Verification items for the finished model (mm, model axes). Face numbers are marked on the shaded views. A direction names the side the tool comes from. Coordinates: 2 decimals unless noted, no trailing zeros. Loops run counter-clockwise (first coordinate to the right, second up) from the corner with the lowest first, then second, coordinate; pieces in that order, holes last.
Q1. Sectioned sample at B-B (y = 155.5). Enter the section's corners in (x, z).
Q2. Mould release check, pull along X, two halves, no side actions. Record for the marked faces 3 and 4: +X half, -X half, draft (parallel to the pull), parting line (faces both ways), or undercut.
Q3. Sectioned sample at A-A (x = 57). Enter the section's corners in (y, z), then the cut area to 3 significant figures.
Q4. Material ranges on probe 1 along X at (y, z) = (9, 7.5); probe 2 along Y at (x, z) = (20, 3.75); probe 3 along Y at (x, z) = (79, 9), recorded low to high.
Q5. Go/stop test with flat-tipped pins: P1, Ø7.5, axis at x = 66, z = 5, coming from the +Y side; P2, Ø4.5, axis at x = 130, z = 7.5, coming from the +Y side; P3, Ø6, axis at x = 80, z = 7.5, coming from the +Y side. Record where each tip stops, or that it passes through.
Q6. Access from +Z, -Z, +X, -X, +Y, -Y to the whole of each face (thin tool, end or side, straight path). Record for the marked faces 1 and 2.
Q7. Sectioned sample at C-C (y = 178). Enter the section's corners in (x, z), then the cut area to 3 significant figures.
```python
from build123d import *

# Parameters (mm, degrees)
EXTRUDE_1_DEPTH        = 15
CUT_EXTRUDE_1_DEPTH    = 267.118858915
FILLET_1_R             = 10
PATTERN_LINEAR_1_COUNT = 3
PATTERN_LINEAR_1_PITCH = 50
PATTERN_LINEAR_2_COUNT = 3
PATTERN_LINEAR_2_PITCH = 80
HOLE_WIZARD_M6_3_D     = 5


with BuildPart() as part:
    # 草图1 → 凸台-拉伸1 (new body)
    with BuildSketch(Plane.XY):
        Polygon((0, 0), (163.629943485, 0), (163.629943485, 94.33), (0, 209.331050409), align=None)
    extrude(amount=EXTRUDE_1_DEPTH)

    # 草图2 → 切除-拉伸1 (cut, through all)
    with BuildSketch(Plane.XY.offset(15)):
        Polygon((25, 161.2040017), (25, 25), (138.629943485, 25), (138.629943485, 81.343539854), align=None)
    extrude(amount=-CUT_EXTRUDE_1_DEPTH, mode=Mode.SUBTRACT)

    # 圆角1
    fillet_1_edges = [part.edges().sort_by_distance(p)[0] for p in [
        (25, 161.2040017, 7.5),
        (138.629943485, 81.343539854, 7.5),
        (138.629943485, 25, 7.5),
        (25, 25, 7.5),
    ]]
    fillet(fillet_1_edges, radius=FILLET_1_R)

    # 草图3 → M6 螺纹孔1 (revolve, cut)
    with BuildSketch(Plane(origin=(30, 0, 7.5), x_dir=(0, 0, -1), z_dir=(1, 0, 0))):
        Polygon((0, 0), (0, 16.502151548), (2.5, 15), (2.5, 0), align=None)
    hole_wizard_m6_1 = revolve(axis=Axis((30, -6.35, 7.5), (0, 1, 0)), mode=Mode.SUBTRACT)

    # 阵列(线性)1: M6 螺纹孔1 ×3
    with Locations(*[(i * PATTERN_LINEAR_1_PITCH, 0, 0) for i in range(1, PATTERN_LINEAR_1_COUNT)]):
        add(hole_wizard_m6_1, mode=Mode.SUBTRACT)

    # 草图5 → M6 螺纹孔2 (revolve, cut)
    with BuildSketch(Plane(origin=(147.266949137, 105.830105041, 7.5), x_dir=(-0.8181497174250246, 0.5750052520432769, 0), z_dir=(0, 0, 1))):
        Polygon((0, 0), (0, 16.502151548), (2.5, 15), (2.5, 0), align=None)
    hole_wizard_m6_2 = revolve(axis=Axis((150.918232487, 111.025355747, 7.5), (-0.5750052520432769, -0.8181497174250246, 0)), mode=Mode.SUBTRACT)

    # 阵列(线性)2: M6 螺纹孔2 ×3
    with Locations(*[Vector(-0.8181497174250245, 0.575005252043277, 0) * (i * PATTERN_LINEAR_2_PITCH) for i in range(1, PATTERN_LINEAR_2_COUNT)]):
        add(hole_wizard_m6_2, mode=Mode.SUBTRACT)

    # M6 螺纹孔3 (through all)
    with Locations(Plane.XY.offset(15)):
        with Locations((20, 27), (20, 52), (10, 52), (10, 27), (143.629943485, 52), (153.629943485, 52), (143.629943485, 27), (153.629943485, 27)):
            Hole(HOLE_WIZARD_M6_3_D / 2)


solid = part.part
```
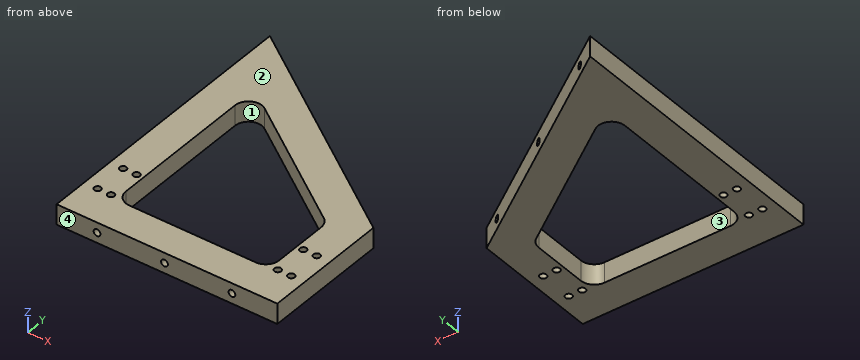
Geometry check:
1. outline: (0, 0) - (76.59, 0) - (76.59, 15) - (0, 15) - close
2. face 3: undercut
2. face 4: draft
3. outline: (0, 0) - (25, 0) - (25, 15) - (0, 15) - close; (138.71, 0) - (169.27, 0) - (169.27, 15) - (138.71, 15) - close
3. area: 833 mm2
4. probe 1: x = 0 to 27.5, 32.5 to 77.5, 82.5 to 127.5, 132.5 to 163.63
4. probe 2: y = 0 to 24.5, 29.5 to 49.5, 54.5 to 195.27
4. probe 3: y = 15.42 to 25, 123.25 to 144.35, 151.3 to 153.81
5. P1: stops at y = 165.58
5. P2: stops at y = 119.55
5. P3: stops at y = 155.21
6. face 1: +Z, -Z
6. face 2: +Z, +X, -X, +Y, -Y
7. outline: (0, 0) - (44.58, 0) - (44.58, 15) - (0, 15) - close
7. area: 669 mm2
